Source: CAD feature listing. Evaluate the final solid. Frame: model axes, mm. A direction names the side the tool comes from. Coordinates: 2 decimals unless noted, no trailing zeros. Order: outer loops, then holes, each group sorted by start corner. A loop starts at its lowest first (then second) coordinate and runs counter-clockwise, first axis right, second up.
```python
from build123d import *

# Parameters (mm, degrees)
SKETCH1_R           = 1
BOSS_EXTRUDE5_DEPTH = 1
SKETCH3_R           = 1
BOSS_EXTRUDE6_DEPTH = 0.5
SKETCH5_R           = 1
BOSS_EXTRUDE8_DEPTH = 1
SKETCH6_R           = 1
BOSS_EXTRUDE9_DEPTH = 1


with BuildPart() as part:
    # Sketch1 → Boss-Extrude5 (new body)
    with BuildSketch(Plane(origin=(0, 0, 0), x_dir=(1, 0, 0), z_dir=(0, 1, 0))):
        with BuildLine():
            Line((-47.682880055, 11.164224632), (-47.682880055, -8.835775368))
            ThreePointArc((-47.682880055, -8.835775368), (-46.828715239, -10.932294236), (-44.752619147, -11.834964669))
            Line((-44.752619147, -11.834964669), (4.512839673, -2.999578636))
            ThreePointArc((4.512839673, -2.999578636), (7.487489348, 0.025350325), (4.462560387, 3))
            Line((4.462560387, 3), (-43.657583095, 13.983580257))
            ThreePointArc((-43.657583095, 13.983580257), (-46.403942099, 13.621447747), (-47.682880055, 11.164224632))
        make_face()
        with Locations((-44.682880055, 11.164224632)):
            Circle(SKETCH1_R, mode=Mode.SUBTRACT)
        with Locations((-44.682880055, -8.835775368)):
            Circle(SKETCH1_R, mode=Mode.SUBTRACT)
        with Locations((4.462560387, 0)):
            Circle(SKETCH1_R, mode=Mode.SUBTRACT)
    extrude(amount=BOSS_EXTRUDE5_DEPTH)

    # Sketch3 → Boss-Extrude6 (add, symmetric)
    with BuildSketch(Plane(origin=(0, 1, 0), x_dir=(1, 0, 0), z_dir=(0, 1, 0))):
        with Locations((4.462560387, 0)):
            Circle(SKETCH3_R)
    extrude(amount=BOSS_EXTRUDE6_DEPTH, both=True)

    # Sketch5 → Boss-Extrude8 (add)
    with BuildSketch(Plane(origin=(0, 1, 0), x_dir=(1, 0, 0), z_dir=(0, 1, 0))):
        with Locations((4.462560387, 0)):
            Circle(SKETCH5_R)
    extrude(amount=BOSS_EXTRUDE8_DEPTH)

    # Sketch6 → Boss-Extrude9 (add, symmetric)
    with BuildSketch(Plane(origin=(0, 1, 0), x_dir=(1, 0, 0), z_dir=(0, 1, 0))):
        with Locations((-44.682880055, -8.835775368)):
            Circle(SKETCH6_R)
    extrude(amount=BOSS_EXTRUDE9_DEPTH, both=True)


solid = part.part
```
1. Section query B-B on x = -27.5. Return loops of the section in (y, z).
Findings:
outline: (0, -10.3) - (1, -10.3) - (1, 8.74) - (0, 8.74) - close
2. Pin query (flat end, axial travel): P1, Ø2.5, axis at x = 4.46, z = 0, coming from the -Y side; P2, Ø2, axis at x = -26.5, z = -11, coming from the +Y side. Return the tip coordinate at first contact, or that it passes through.
Findings:
P1: stops at y = 0
P2: stops at y = 1
3. Section query A-A on z = 0. Return loops of the section in (x, y), plus the area to 3 significant figures.
Findings:
outline: (-47.68, 0) - (3.46, 0) - (3.46, 0.5) - (5.46, 0.5) - (5.46, 0) - (7.49, 0) - (7.49, 1) - (5.46, 1) - (5.46, 2) - (3.46, 2) - (3.46, 1) - (-47.68, 1) - close
area: 56.2 mm2
4. Draft query along X for faces 3 (the face through (4, 2, 0)), 4 (the face through (-46.85, 0.49, 10.91)), 5 (the face through (-45.42, 1.51, 8.16)), 6 (the face through (-45.68, 0.49, -11.21)). Return one class per face: released by +X, released by -X, zero draft, split by the parting line, or undercut.
Findings:
face 3: zero draft
face 4: released by -X
face 5: split by the parting line
face 6: undercut
5. Ray query, line 1 (X direction, y = 0.2, z = 0); line 2 (Y direction, x = -44, z = -2.75); line 3 (Z direction, x = 1, y = 0.65). Return the intervals inside material, ascending.
Findings:
line 1: x = -47.68 to 3.46, 5.46 to 7.49
line 2: y = 0 to 1
line 3: z = -3.79 to 3.63
6. Section query C-C on x = 2. Return loops of the section in (y, z).
Findings:
outline: (0, -3.56) - (1, -3.56) - (1, 3.45) - (0, 3.45) - close
7. Access query for faces 1 (the face through (4, 0.5, 0)), 2 (the face through (-47.683, 0.5, -1.3)). Directions: +Z, -Z, +X, -X, +Y, -Y. A direction counts if a zero-diameter tool reaches every point of the face in a straight line with its end or side. Return the directions, or none.
Findings:
face 1: -Y
face 2: +Z, -Z, -X, +Y, -Y
